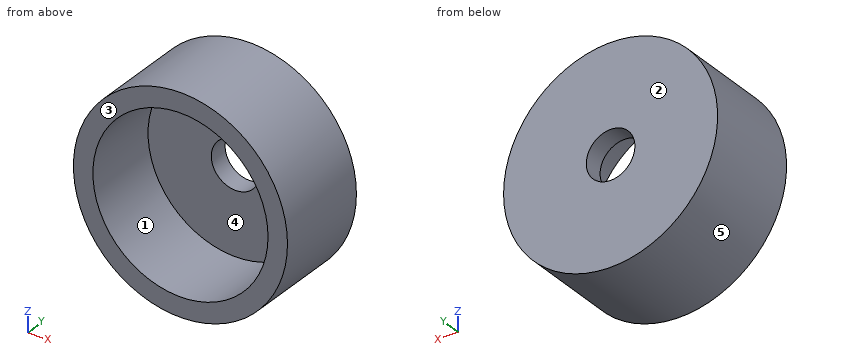
from build123d import *

# Parameters (mm, degrees)
F0_R     = 11
F1_DEPTH = 2
F2_R     = 2.5
F3_DEPTH = 25
F4_R     = 11
F4_R_2   = 9
F5_DEPTH = 8


with BuildPart() as f1:
    # F0 (on Front) → F1 (new body)
    with BuildSketch(Plane.XZ):
        Circle(F0_R)
    extrude(amount=F1_DEPTH)

    # F2 (on face) → F3 (cut)
    with BuildSketch(Plane.XZ.offset(2)):
        Circle(F2_R)
    extrude(amount=-F3_DEPTH, mode=Mode.SUBTRACT)

    # F4 (on face) → F5 (join)
    with BuildSketch(Plane.XZ.offset(2)):
        Circle(F4_R)
        Circle(F4_R_2, mode=Mode.SUBTRACT)
    extrude(amount=F5_DEPTH)


solid = f1.part
Read the model definition and answer for the solid it produces. Units are mm, in the model's axes. Face numbers are marked on the shaded views. A direction names the side the tool comes from. Coordinates: 2 decimals unless noted, no trailing zeros. Loops run counter-clockwise (first coordinate to the right, second up) from the corner with the lowest first, then second, coordinate; pieces in that order, holes last. Notation, with made-up numbers: (32.25, -13.75) - (48.25, -13.75) arc R22 cw to (48.25, 10.25) - close; hole circle Ø10 at (35.5, -23). An arc over 180 degrees is marked (long way). Answer in a Markdown table with one row per item.
Q1. Straight lines are drawn through the part: line 1 along Z through (x, y) = (0, -5.5); line 2 along Z through (x, y) = (0, -1.6); line 3 along Y through (x, z) = (-3, -3.25). For each, find the intervals that lie inside material, in ascending order. Write a range as [from, to].
Here are the results:
| item | result |
|---|---|
| line 1 | z = [-11, -9], [9, 11] |
| line 2 | z = [-11, -2.5], [2.5, 11] |
| line 3 | y = [-2, 0] |
Q2. Find section D-D on z = 3.5. Write down the section's boundary in (x, y).
Here are the results:
| item | result |
|---|---|
| outline | (-10.43, -10) - (-8.29, -10) - (-8.29, -2) - (8.29, -2) - (8.29, -10) - (10.43, -10) - (10.43, 0) - (-10.43, 0) - close |
Q3. Find section B-B on z = 0. Write down the section's boundary in (x, y).
Here are the results:
| item | result |
|---|---|
| outline | (-11, -10) - (-9, -10) - (-9, -2) - (-2.5, -2) - (-2.5, 0) - (-11, 0) - close; (2.5, -2) - (9, -2) - (9, -10) - (11, -10) - (11, 0) - (2.5, 0) - close |
Q4. Find section A-A on x = 0. Write down the section's boundary in (y, z).
Here are the results:
| item | result |
|---|---|
| outline | (-10, -11) - (0, -11) - (0, -2.5) - (-2, -2.5) - (-2, -9) - (-10, -9) - close; (-10, 9) - (-2, 9) - (-2, 2.5) - (0, 2.5) - (0, 11) - (-10, 11) - close |
Q5. The mould has two halves that part along Z. Classify the marked faces 3, 4 and 5: pulls with the +Z half, pulls with the -Z half, needs draft (parallel to the pull), parting line crosses it, or undercut.
Here are the results:
| item | result |
|---|---|
| face 3 | needs draft |
| face 4 | undercut |
| face 5 | parting line crosses it |
Q6. Find section C-C on y = -8.5. Write down the section's boundary in (x, z), plus the area to 3 significant figures.
Here are the results:
| item | result |
|---|---|
| outline | circle Ø22 at (0, 0); hole circle Ø18 at (0, 0) |
| area | 126 mm^2 |
Q7. Given P1, Ø1.5, axis at y = -7.5, z = 6, coming from the +X side; P2, Ø4, axis at x = -8, y = -8.5, coming from the -Z side; P3, Ø8, axis at x = -2, z = -2, coming from the -Y side; P4, Ø4.5, axis at x = 0, z = 0, coming from the -Y side, each flat-ended and moving along its own axis, determine where each tip first touches the part or whether it passes through.
Here are the results:
| item | result |
|---|---|
| P1 | stops at x = 9.67 |
| P2 | stops at z = -9.22 |
| P3 | stops at y = -2 |
| P4 | passes through |
Q8. For the marked faces 1 and 2, determine the directions among +Z, -Z, +X, -X, +Y, -Y from which every point of the face is accessible in a straight line to the end or side of a thin tool.
Here are the results:
| item | result |
|---|---|
| face 1 | -Y |
| face 2 | +Z, -Z, +X, -X, +Y |
